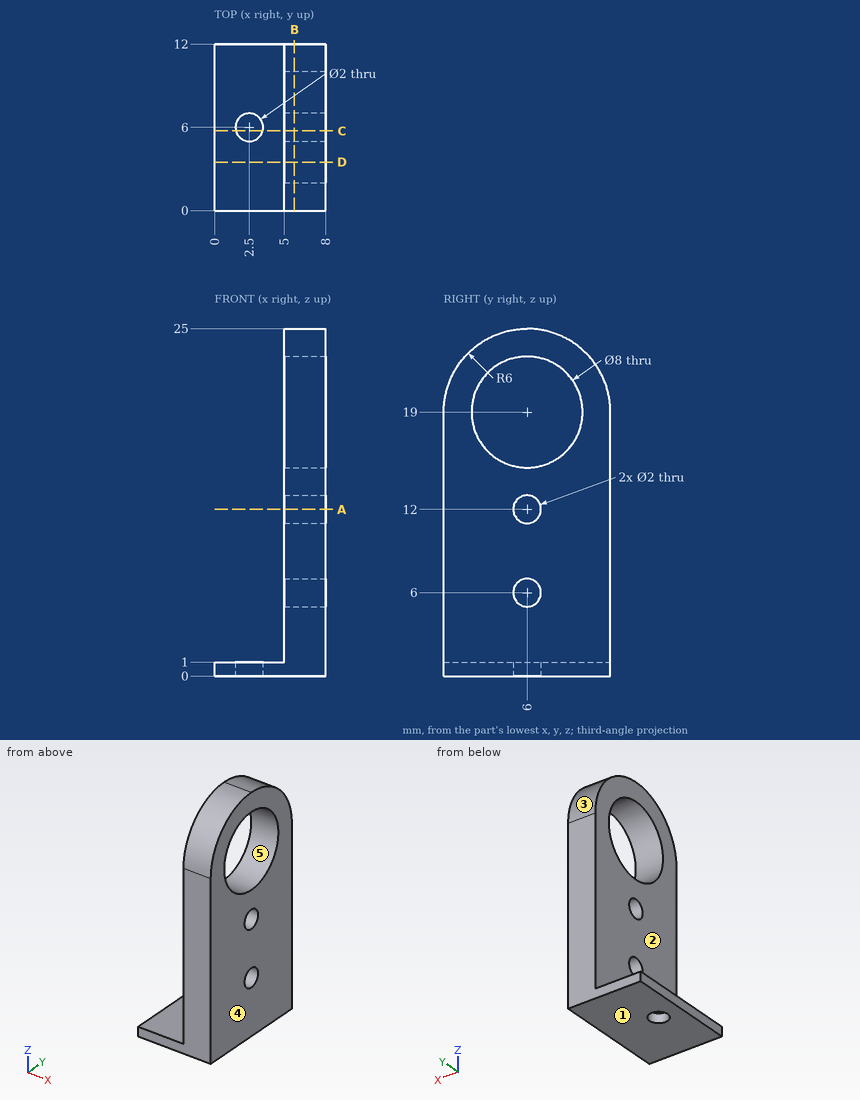
Answer from the drawing. Dimensions are ordinates in mm from the lowest x, y and z of the part. A direction names the side the tool comes from. Give positions to 0.01 mm unless a question says otherwise; leave off trailing zeros. Write each loop counter-clockwise with the first axis right and the second up, starting at its lowest first coordinate (ties: lowest second). Pieces come first, ordered by that corner, then holes. Notation, with made-up numbers: (64.5, 68.5) - (71.5, 68.5) arc R16 ccw to (71.5, 89.5) - close; hole circle Ø11 at (65.5, 19.25). An arc over 180 degrees is marked (long way). Answer in a Markdown table with one row per item. Add a question column.
Item 1: Section B-B, the plane x = 5.75 is taken. Count the separate pieces of the cut face and the enclosed holes in it, and give its area (3 significant figures).
Item 2: A flat-ended cylindrical pin translates along its axis: P1, Ø3, axis at y = 6, z = 6, coming from the -X side. Find the tip coordinate at first contact, or state that the pin passes through.
Item 3: Determine the mould class of the marked faces 3, 4 and 5 for opening direction Y: pulls with the +Y half, pulls with the -Y half, needs draft (parallel to the pull), parting line crosses it, or undercut.
Item 4: Section A-A, the plane z = 12 is taken. Write down the section's boundary in (x, y).
Item 5: Section D-D, the plane y = 3.5 is taken. Write down the section's boundary in (x, z), and give its area (3 significant figures).
Item 6: Section C-C, the plane y = 5.75 is taken. Write down the section's boundary in (x, z).
Item 7: A tool of negligible diameter and unlimited length cuts with its end or side. For the marked faces 1 and 2, from which of +Z, -Z, +X, -X, +Y, -Y can it reach the whole face along a straight path? Write none if from no direction.
Item 8: Find the intervals of material crossed by L1, parallel to Z at x = 6.05, y = 6; L2, parallel to Y at x = 2.5, z = 0.25; L3, parallel to Z at x = 4, y = 0.5, in increasing order.
Recorded:
| question | item | result |
|---|---|---|
| 1 | separate pieces | 1 |
| 1 | enclosed holes | 3 |
| 1 | area | 228 mm2 |
| 2 | P1 | stops at x = 5 |
| 3 | face 3 | pulls with the +Y half |
| 3 | face 4 | needs draft |
| 3 | face 5 | undercut |
| 4 | outline | (5, 0) - (8, 0) - (8, 5) - (5, 5) - close; (5, 7) - (8, 7) - (8, 12) - (5, 12) - close |
| 5 | outline | (0, 0) - (8, 0) - (8, 15.88) - (5, 15.88) - (5, 1) - (0, 1) - close; (5, 22.12) - (8, 22.12) - (8, 24.45) - (5, 24.45) - close |
| 5 | area | 59.6 mm2 |
| 6 | outline | (0, 0) - (1.53, 0) - (1.53, 1) - (0, 1) - close; (3.47, 0) - (8, 0) - (8, 5.03) - (5, 5.03) - (5, 1) - (3.47, 1) - close; (5, 6.97) - (8, 6.97) - (8, 11.03) - (5, 11.03) - close; (5, 12.97) - (8, 12.97) - (8, 15.01) - (5, 15.01) - close; (5, 22.99) - (8, 22.99) - (8, 24.99) - (5, 24.99) - close |
| 7 | face 1 | -Z, +X, -X, +Y, -Y |
| 7 | face 2 | +Z, -X, +Y, -Y |
| 8 | L1 | z = 0 to 5, 7 to 11, 13 to 15, 23 to 25 |
| 8 | L2 | y = 0 to 5, 7 to 12 |
| 8 | L3 | z = 0 to 1 |
